```python
from build123d import *

# Parameters (mm, degrees)
F1_DEPTH = 35
F2_DEPTH = 2
F3_W     = 9
F3_H     = 11
F4_DEPTH = 3
F5_R     = 12.5
F6_DEPTH = 130
F7_R     = 10.5
F8_DEPTH = 3


with BuildPart() as f1:
    # F0 (on Top) → F1 (new body)
    with BuildSketch(Plane.XY):
        Polygon((0.0621920733, 62.8993051266), (-44.1054810761, 45.2816312037), (-63.2062332438, 0.831663731), (-45.2816312037, -44.1054810761), (-0.831663731, -63.2062332438), (43.3360094184, -45.5885593209), (61.7826262379, -2.6608510081), (42.9899003861, 44.4526883072), align=None)
        Polygon((-42.9555200118, -41.8397885551), (-59.9593377004, 0.788941279), (-41.8397885551, 42.9555200118), (0.0194696214, 59.6524095833), (40.6637891941, 42.1869957861), (58.5357306946, -2.6181285562), (41.0703168974, -43.2624481289), (-0.788941279, -59.9593377004), align=None, mode=Mode.SUBTRACT)
    extrude(amount=F1_DEPTH)

    # F0 (on Top) → F2 (join)
    with BuildSketch(Plane.XY):
        Polygon((-41.8397885551, 42.9555200118), (-59.9593377004, 0.788941279), (-42.9555200118, -41.8397885551), (-0.788941279, -59.9593377004), (41.0703168974, -43.2624481289), (58.5357306946, -2.6181285562), (40.6637891941, 42.1869957861), (0.0194696214, 59.6524095833), align=None)
    extrude(amount=F2_DEPTH)

    # F3 (on face) → F4 (cut, through all)
    with BuildSketch(Plane(origin=(53.1176572725, -22.8253756971, 0), x_dir=(0.3948056073, 0.9187646774, 0), z_dir=(0.9187646774, -0.3948056073, 0))):
        with Locations((-1.2642135624, 11.5)):
            Rectangle(F3_W, F3_H)
    extrude(amount=-F4_DEPTH, mode=Mode.SUBTRACT)

    # F5 (on face) → F6 (join)
    with BuildSketch(Plane.XY.offset(2)):
        Circle(F5_R)
    extrude(amount=F6_DEPTH)

    # F7 (on face) → F8 (cut, through all)
    with BuildSketch(Plane(origin=(-53.6558571599, 23.0566474674, 0), x_dir=(-0.3948056073, -0.9187646774, 0), z_dir=(-0.9187646774, 0.3948056073, 0))):
        with Locations((0, 17.5)):
            Circle(F7_R)
    extrude(amount=-F8_DEPTH, mode=Mode.SUBTRACT)


solid = f1.part
```
Geometry: final body of the model. Coordinates: model frame, mm. A direction names the side the tool comes from. Coordinates: 2 decimals unless noted, no trailing zeros. Order: outer loops, then holes, each group sorted by start corner. A loop starts at its lowest first (then second) coordinate and runs counter-clockwise, first axis right, second up. Notation, with made-up numbers: M -39,77.25 L -32,77.25 A21 cw -32,88.25 Z; hole C 76.25,64 d1. An arc over 180 degrees is marked long. Answer in a Markdown table with one row per item. Add a question column.
Q1. Mould query, pull axis X, two halves, no side actions, for faces 3 (the flat face through (-52, -23, 35)), 4 (the flat face through (-49.278, 33.246, 17.255)), 5 (the cylindrical face through (-51.76, 23.73, 27.91)), 6 (the flat face through (52.43, -24.43, 17.26)). Classes: released by +X, released by -X, zero draft, split by the parting line, or undercut.
Q2. Reachability of faces 1 (the flat face through (-23.37, -53.52, 17.26)), 2 (the flat face through (-21.577, -51.026, 18.269)) from +Z, -Z, +X, -X, +Y, -Y: full face, straight path, thin tool, end or side. Return the list, or none.
Q3. Section query B-B on x = 36. Return the cut outline in (y, z), and give its area (3 significant figures).
Q4. Section query D-D on z = 60. Return the cut outline in (x, y), and give its area (3 significant figures).
Q5. Section query A-A on z = 9.5. Return the cut outline in (x, y).
Q6. Contact query for flat-ended pins moving along their axis: P1, Ø3, axis at y = -12.5, z = 30, coming from the -X side; P2, Ø5, axis at x = 13.5, z = 84, coming from the +Y side; P3, Ø3, axis at x = 53, y = -23, coming from the +Z side. Output: stop coordinate, or through.
Q7. Section query C-C on y = -54.5. Return the cut outline in (x, z).
Q8. Line query: L1, parallel to Y at x = 11, z = 16; L2, parallel to Z at x = -43.5, y = -42; L3, parallel to Y at x = -42.5, z = 7. Output: solid intervals per line, ascending.
Completed:
| question | item | result |
|---|---|---|
| 1 | face 3 | zero draft |
| 1 | face 4 | released by -X |
| 1 | face 5 | undercut |
| 1 | face 6 | released by +X |
| 2 | face 1 | +Z, -Z, -X, -Y |
| 2 | face 2 | +Z |
| 3 | outline | M -48.51,0 L 47.46,0 L 47.46,35 L 44.19,35 L 44.19,2 L -45.28,2 L -45.28,35 L -48.51,35 Z |
| 3 | area | 406 mm2 |
| 4 | outline | C 0,0 d25 |
| 4 | area | 491 mm2 |
| 5 | outline | M -63.21,0.83 L -45.28,-44.11 L -0.83,-63.21 L 43.34,-45.59 L 50.84,-28.12 L 48.09,-26.94 L 41.07,-43.26 L -0.79,-59.96 L -42.96,-41.84 L -59.96,0.79 L -53.58,15.62 L -56.34,16.81 Z; M -50.97,29.3 L -48.21,28.12 L -41.84,42.96 L 0.02,59.65 L 40.66,42.19 L 58.54,-2.62 L 51.64,-18.67 L 54.4,-19.85 L 61.78,-2.66 L 42.99,44.45 L 0.06,62.9 L -44.11,45.28 Z; C 0,0 d25 |
| 6 | P1 | stops at x = -58.49 |
| 6 | P2 | stops at y = 5.94 |
| 6 | P3 | stops at z = 35 |
| 7 | outline | M -21.09,0 L 20.99,0 L 20.99,35 L 12.9,35 L 12.9,2 L -13.49,2 L -13.49,35 L -21.09,35 Z |
| 8 | L1 | y = -58.49 to -55.26, -5.94 to 5.94, 54.93 to 58.2 |
| 8 | L2 | z = 0 to 35 |
| 8 | L3 | y = -45.3 to -42.04, 41.42 to 45.92 |
